from build123d import *

# Parameters (mm, degrees)
SKETCH1_R           = 4
BOSS_EXTRUDE1_DEPTH = 50
SKETCH2_R           = 5
BOSS_EXTRUDE2_DEPTH = 3
SKETCH3_R           = 4
BOSS_EXTRUDE3_DEPTH = 10
SKETCH4_R           = 5
BOSS_EXTRUDE4_DEPTH = 3
SKETCH5_R           = 4
BOSS_EXTRUDE5_DEPTH = 34


with BuildPart() as part:
    # Sketch1 → Boss-Extrude1 (new body)
    with BuildSketch(Plane.XY):
        Circle(SKETCH1_R)
    extrude(amount=BOSS_EXTRUDE1_DEPTH)

    # Sketch2 → Boss-Extrude2 (add)
    with BuildSketch(Plane(origin=(0, 0, 0), x_dir=(-1, 0, 0), z_dir=(0, 0, -1))):
        Circle(SKETCH2_R)
    extrude(amount=BOSS_EXTRUDE2_DEPTH)

    # Sketch3 → Boss-Extrude3 (add)
    with BuildSketch(Plane(origin=(0, 0, -3), x_dir=(-1, 0, 0), z_dir=(0, 0, -1))):
        Circle(SKETCH3_R)
    extrude(amount=BOSS_EXTRUDE3_DEPTH)

    # Sketch4 → Boss-Extrude4 (add)
    with BuildSketch(Plane(origin=(0, 0, -13), x_dir=(-1, 0, 0), z_dir=(0, 0, -1))):
        Circle(SKETCH4_R)
    extrude(amount=BOSS_EXTRUDE4_DEPTH)

    # Sketch5 → Boss-Extrude5 (add)
    with BuildSketch(Plane(origin=(0, 0, -16), x_dir=(-1, 0, 0), z_dir=(0, 0, -1))):
        Circle(SKETCH5_R)
    extrude(amount=BOSS_EXTRUDE5_DEPTH)


solid = part.part
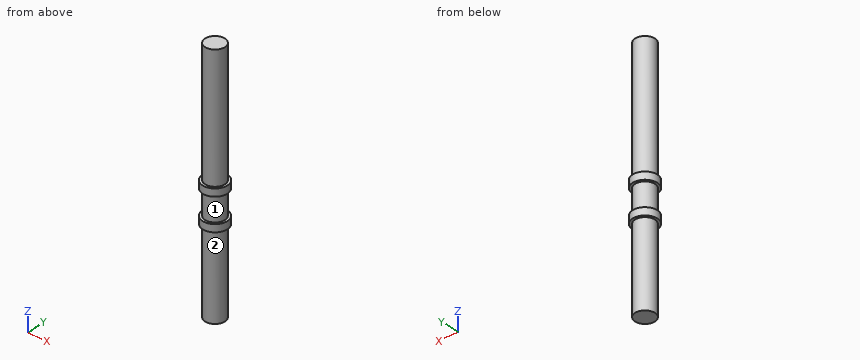
Can you work these out from the model? Positions are in its coordinate system, mm. Face numbers are marked on the shaded views. Give positions to 0.01 mm unless a question says otherwise; leave off trailing zeros. Loops run counter-clockwise (first coordinate to the right, second up) from the corner with the lowest first, then second, coordinate; pieces in that order, holes last. Notation, with made-up numbers: (63.25, 68.5) - (106.25, 68.5) arc R35 ccw to (106.25, 106.5) - close; hole circle Ø4 at (7, -10). An arc over 180 degrees is marked (long way). Answer as a JSON object with one key per item and string values.
Q1. If we mould it in two halves opening along Z, with no side actions, what happens to the marked faces 1 and 2? For each: pulls with the +Z half, pulls with the -Z half, needs draft (parallel to the pull), parting line crosses it, or undercut.
Geometry says:
{"face 1": "undercut", "face 2": "needs draft"}
Q2. Imagine slicing it at A-A on y = 0. Write out the boundary of the cut face in (x, z), plus the area to 3 significant figures.
Geometry says:
{"outline": "(-5, -16) - (-4, -16) - (-4, -50) - (4, -50) - (4, -16) - (5, -16) - (5, -13) - (4, -13) - (4, -3) - (5, -3) - (5, 0) - (4, 0) - (4, 50) - (-4, 50) - (-4, 0) - (-5, 0) - (-5, -3) - (-4, -3) - (-4, -13) - (-5, -13) - close", "area": "812 mm²"}
Q3. Imagine slicing it at C-C on z = 27. Write out the boundary of the cut face in (x, y).
Geometry says:
{"outline": "circle Ø8 at (0, 0)"}
Q4. Will these pins go through, and if not, where does the flat tip stop? P1, Ø4, axis at x = 2.5, z = 39.5, coming from the -Y side; P2, Ø6, axis at y = -2, z = -25.5, coming from the +X side.
Geometry says:
{"P1": "y = -3.97", "P2": "x = 4"}
Q5. If I drill on L1, parallel to Z at x = -3.5, y = -2.75; L2, parallel to X at y = 0.25, z = 21; L3, parallel to X at y = 1.25, z = 10.5, over which ranges is the centre line in solid material (lowest first)?
Geometry says:
{"L1": "-16 to -13, -3 to 0", "L2": "-3.99 to 3.99", "L3": "-3.8 to 3.8"}
